from build123d import *

# Parameters (mm, degrees)
F0_W     = 30
F0_H     = 30
F0_W_2   = 24
F0_H_2   = 24
F1_DEPTH = 500
F3_DEPTH = 30.001


with BuildPart() as f1:
    # F0 (on Front) → F1 (new body)
    with BuildSketch(Plane.XZ):
        Rectangle(F0_W, F0_H)
        Rectangle(F0_W_2, F0_H_2, mode=Mode.SUBTRACT)
    extrude(amount=F1_DEPTH)

    # F2 (on face) → F3 (cut, through all)
    with BuildSketch(Plane(origin=(0, 0, -15), x_dir=(1, 0, 0), z_dir=(0, 0, -1))):
        Polygon((-15, 380.188794), (15, 369.269687), (15, 500), (-15, 500), align=None)
        Polygon((-15, 0), (15, 0), (-15, 10.919107), align=None)
    extrude(amount=-F3_DEPTH, mode=Mode.SUBTRACT)


solid = f1.part
Source: CAD feature listing. Evaluate the final solid. Frame: model axes, mm. A direction names the side the tool comes from. Coordinates: 2 decimals unless noted, no trailing zeros. Loops run counter-clockwise (first coordinate to the right, second up) from the corner with the lowest first, then second, coordinate; pieces in that order, holes last. Notation, with made-up numbers: (-11, 70) - (15, 70) arc R24 cw to (15, 84) - close; hole circle Ø11 at (1.5, 30). An arc over 180 degrees is marked (long way). One line per question, with ' | ' between items.
1) Section C-C, the plane x = -8. Return loops of the section in (y, z).
Report:
outline: (-377.64, -15) - (-8.37, -15) - (-8.37, -12) - (-377.64, -12) - close; (-377.64, 12) - (-8.37, 12) - (-8.37, 15) - (-377.64, 15) - close
2) Pull-direction query (Z, two-part tool) for faces 1 (the face through (0, -187, -15)), 2 (the face through (-12, -192, 0)), 3 (the face through (0, -187, 15)); classes: released by +Z, released by -Z, zero draft, split by the parting line, or undercut.
Report:
face 1: released by -Z | face 2: undercut | face 3: released by +Z
3) Line query: line 1 along Z through (x, y) = (2.5, -140.5); line 2 along Y through (x, z) = (-12.5, 12). Output: solid intervals per line, ascending.
Report:
line 1: z = -15 to -12, 12 to 15 | line 2: y = -379.28 to -10.01
4) Section A-A, the plane z = 6. Return loops of the section in (x, y), then the cut area to 3 significant figures.
Report:
outline: (-15, -380.19) - (-12, -379.1) - (-12, -9.83) - (-15, -10.92) - close; (12, -370.36) - (15, -369.27) - (15, 0) - (12, -1.09) - close | area: 2,220 mm²
5) Set-up query: faces 4 (the face through (0, -187, -12)), 5 (the face through (-15, -193, 0)). Return all of +Z, -Z, +X, -X, +Y, -Y with unobstructed straight access to the full face (end or side cutting, diameter ignored); none if empty.
Report:
face 4: +Y, -Y | face 5: +Z, -Z, -X, +Y, -Y
6) Section B-B, the plane y = -220.5. Return loops of the section in (x, z), then the cut area to 3 significant figures.
Report:
outline: (-15, -15) - (15, -15) - (15, 15) - (-15, 15) - close; hole (-12, -12) - (12, -12) - (12, 12) - (-12, 12) - close | area: 324 mm²
